from build123d import *

# Parameters (mm, degrees)
CHANNEL_DEPTH             = 39.35
CHANNEL_DEPTH_BACK        = 19.15
FLANGES_SKETCH_W          = 8.6
FLANGES_SKETCH_H          = 3
FLANGES_DEPTH             = 10.6
SERVO_HOLES_SKETCH_R      = 1.6
SERVO_HOLES_DEPTH         = 54.2
PANEL_HOLE_SKETCH_R       = 10.05
PANEL_HOLE_DEPTH          = 16.4
PANEL_NUT_RELIEF_SKETCH_W = 14.5
PANEL_NUT_RELIEF_SKETCH_H = 5


with BuildPart() as part:
    # Channel Sketch → Channel (new, two sides: drawn at the far end of the back side and taken through both)
    with BuildSketch(Plane(origin=(0, 0, 0), x_dir=(0, 0, -1), z_dir=(1, 0, 0)).offset(-CHANNEL_DEPTH_BACK)):
        Polygon((-12.1, 12.2), (12.1, 12.2), (12.1, 44.2), (10.6, 44.2), (10.6, 15.4), (-10.6, 15.4), (-10.6, 44.2), (-12.1, 44.2), align=None)
    extrude(amount=CHANNEL_DEPTH + CHANNEL_DEPTH_BACK)

    # Flanges Sketch → Flanges (add, symmetric)
    with BuildSketch(Plane.XY):
        with Locations((-14.85, 42.7)):
            Rectangle(FLANGES_SKETCH_W, FLANGES_SKETCH_H)
        with Locations((35.05, 42.7)):
            Rectangle(FLANGES_SKETCH_W, FLANGES_SKETCH_H)
    extrude(amount=FLANGES_DEPTH, both=True)

    # Servo Holes Sketch → Servo Holes (cut, symmetric)
    with BuildSketch(Plane(origin=(0, 0, 0), x_dir=(1, 0, 0), z_dir=(0, 1, 0))):
        with Locations(Location((-14.65, -5, 0), (0, 0, 270))):
            Circle(SERVO_HOLES_SKETCH_R)
        with Locations(Location((-14.65, 5, 0), (0, 0, 270))):
            Circle(SERVO_HOLES_SKETCH_R)
        with Locations(Location((34.85, -5, 0), (0, 0, 270))):
            Circle(SERVO_HOLES_SKETCH_R)
        with Locations(Location((34.85, 5, 0), (0, 0, 270))):
            Circle(SERVO_HOLES_SKETCH_R)
    extrude(amount=SERVO_HOLES_DEPTH, both=True, mode=Mode.SUBTRACT)

    # Panel Hole Sketch → Panel Hole (cut, symmetric)
    with BuildSketch(Plane(origin=(0, 0, 0), x_dir=(1, 0, 0), z_dir=(0, 1, 0))):
        with Locations(Location((0, 0, 0), (0, 0, 270))):
            Circle(PANEL_HOLE_SKETCH_R)
    extrude(amount=PANEL_HOLE_DEPTH, both=True, mode=Mode.SUBTRACT)

    # Panel Nut Relief Sketch → Panel Nut Relief (revolve, cut)
    with BuildSketch(Plane.XY):
        with Locations((7.25, 17.9)):
            Rectangle(PANEL_NUT_RELIEF_SKETCH_W, PANEL_NUT_RELIEF_SKETCH_H)
    revolve(axis=Axis((0, -500, 0), (0, 1, 0)), mode=Mode.SUBTRACT)


solid = part.part
The listing builds one solid part. Answer for the finished solid, in the listing's coordinates (mm). A direction names the side the tool comes from. Give positions to 0.01 mm unless a question says otherwise; leave off trailing zeros. Write each loop counter-clockwise with the first axis right and the second up, starting at its lowest first coordinate (ties: lowest second). Pieces come first, ordered by that corner, then holes.
1) Section C-C (y = 25.5) is taken. Write down the section's boundary in (x, z), and give its area (4 significant figures).
2) For a pull along Y with two mould halves and no side action, classify faces 4 (the face through (10, 44.2, -11)), 5 (the face through (36.436, 42.679, 4.792)), 6 (the face through (10, 30, 10.6)) as pulls with the +Y half, pulls with the -Y half, needs draft (parallel to the pull), parting line crosses it, or undercut.
3) A tool of negligible diameter and unlimited length cuts with its end or side. For faces 1 (the face through (35, 41.2, 0)), 2 (the face through (8.987, 17.935, -11.379)), 3 (the face through (30.75, 43, 0)), from which of +Z, -Z, +X, -X, +Y, -Y can it reach the whole face along a straight path? Write none if from no direction.
4) Given P1, Ø7.5, axis at x = 1.5, z = 3.5, coming from the +Y side; P2, Ø8, axis at x = -6, z = 8, coming from the +Y side, each flat-ended and moving along its own axis, determine where each tip first touches the part or whether it passes through.
5) Section A-A (x = 0) is taken. Write down the section's boundary in (y, z), and give its area (3 significant figures).
6) Find the intervals of material crossed by L1, parallel to X at y = 43.25, z = 5; L2, parallel to Y at x = -16.5, z = 4.25, in increasing order.
7) Section B-B (y = 18.5) is taken. Write down the section's boundary in (x, z), and give its area (3 significant figures).
8) Section D-D (x = 27) is taken. Write down the section's boundary in (y, z), and give its area (3 significant figures).
Response:
1. outline: (-19.15, -12.1) - (39.35, -12.1) - (39.35, -10.6) - (-19.15, -10.6) - close; (-19.15, 10.6) - (39.35, 10.6) - (39.35, 12.1) - (-19.15, 12.1) - close
1. area: 175.5 mm2
2. face 4: pulls with the +Y half
2. face 5: needs draft
2. face 6: undercut
3. face 1: +X, -X
3. face 2: none
3. face 3: +Y
4. P1: passes through
4. P2: stops at y = 44.2
5. outline: (12.2, -12.1) - (15.4, -12.1) - (15.4, -10.05) - (12.2, -10.05) - close; (12.2, 10.05) - (15.4, 10.05) - (15.4, 12.1) - (12.2, 12.1) - close; (20.4, -12.1) - (44.2, -12.1) - (44.2, -10.6) - (20.4, -10.6) - close; (20.4, 10.6) - (44.2, 10.6) - (44.2, 12.1) - (20.4, 12.1) - close
5. area: 84.5 mm2
6. L1: x = -19.15 to -16.25, -13.05 to -10.55, 30.75 to 33.25, 36.45 to 39.35
6. L2: y = 12.2 to 15.4, 41.2 to 44.2
7. outline: (-19.15, -12.1) - (-7.99, -12.1) arc R14.5 cw to (-9.89, -10.6) - (-19.15, -10.6) - close; (-19.15, 10.6) - (-9.89, 10.6) arc R14.5 cw to (-7.99, 12.1) - (-19.15, 12.1) - close; (7.99, -12.1) - (39.35, -12.1) - (39.35, -10.6) - (9.89, -10.6) arc R14.5 cw to start; (7.99, 12.1) arc R14.5 cw to (9.89, 10.6) - (39.35, 10.6) - (39.35, 12.1) - close
7. area: 122 mm2
8. outline: (12.2, -12.1) - (44.2, -12.1) - (44.2, -10.6) - (15.4, -10.6) - (15.4, 10.6) - (44.2, 10.6) - (44.2, 12.1) - (12.2, 12.1) - close
8. area: 164 mm2
